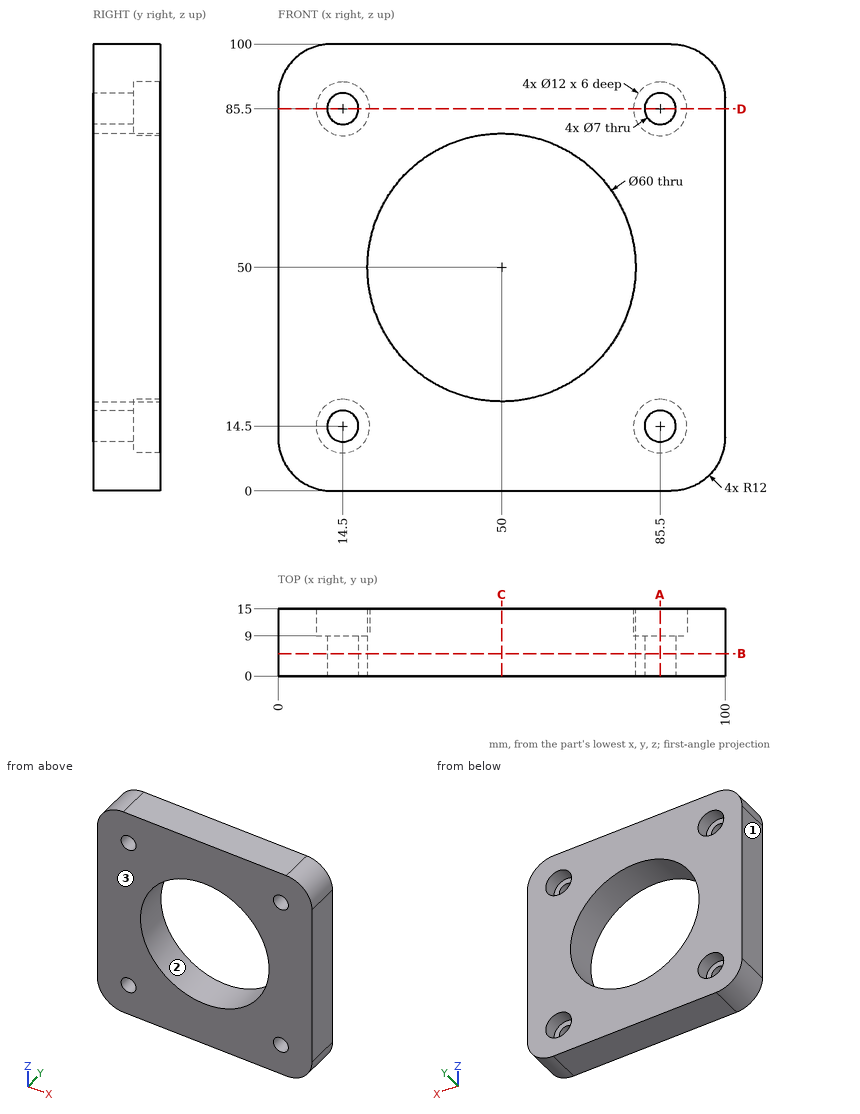
Study the drawing (mm; zero at the part's minimum x, y, z) and answer. Coordinates: 2 decimals unless noted, no trailing zeros. Write each loop counter-clockwise with the first axis right and the second up, starting at its lowest first coordinate (ties: lowest second). Pieces come first, ordered by that corner, then holes. Notation, with made-up numbers: (77.5, 62) - (127.5, 62) arc R16 ccw to (127.5, 89) - close; hole circle Ø3 at (70.5, 60.5). An arc over 180 degrees is marked (long way). One line per item, written item: value.
1) Consider line 1 along X through (y, z) = (10.9, 85.5); line 2 along X through (y, z) = (4.25, 14.5). Determine where each line is inside the solid, lowest interval first. Write a range as from..to.
Geometry check:
line 1: x = 0..8.5, 20.5..79.5, 91.5..100
line 2: x = 0..11, 18..82, 89..100
2) Find section D-D (z = 85.5). Give the vertices of the cut face in (x, y).
Geometry check:
outline: (0, 0) - (11, 0) - (11, 9) - (8.5, 9) - (8.5, 15) - (0, 15) - close; (18, 0) - (82, 0) - (82, 9) - (79.5, 9) - (79.5, 15) - (20.5, 15) - (20.5, 9) - (18, 9) - close; (89, 0) - (100, 0) - (100, 15) - (91.5, 15) - (91.5, 9) - (89, 9) - close
3) For a pull along X with two mould halves and no side action, classify the marked faces 1, 2 and 3 as pulls with the +X half, pulls with the -X half, needs draft (parallel to the pull), parting line crosses it, or undercut.
Geometry check:
face 1: pulls with the -X half
face 2: undercut
face 3: needs draft
4) Find section C-C (x = 50). Give the vertices of the cut face in (y, z).
Geometry check:
outline: (0, 0) - (15, 0) - (15, 20) - (0, 20) - close; (0, 80) - (15, 80) - (15, 100) - (0, 100) - close
5) Find section B-B (y = 5). Give the vertices of the cut face in (x, z), and give its area (4 significant figures).
Geometry check:
outline: (0, 12) arc R12 ccw to (12, 0) - (88, 0) arc R12 ccw to (100, 12) - (100, 88) arc R12 ccw to (88, 100) - (12, 100) arc R12 ccw to (0, 88) - close; hole circle Ø7 at (14.5, 14.5); hole circle Ø7 at (14.5, 85.5); hole circle Ø60 at (50, 50); hole circle Ø7 at (85.5, 14.5); hole circle Ø7 at (85.5, 85.5)
area: 6,895 mm2
6) Find section A-A (x = 85.5). Give the vertices of the cut face in (y, z).
Geometry check:
outline: (0, 0) - (15, 0) - (15, 8.5) - (9, 8.5) - (9, 11) - (0, 11) - close; (0, 18) - (9, 18) - (9, 20.5) - (15, 20.5) - (15, 79.5) - (9, 79.5) - (9, 82) - (0, 82) - close; (0, 89) - (9, 89) - (9, 91.5) - (15, 91.5) - (15, 100) - (0, 100) - close
7) This flat-tipped pin is pushed along its axis until it touches: pin 1 Ø3.5 at (x, z) = (83, 83) entering from +Y. Where does it stop, or does it pass through?
Geometry check:
pin 1: stops at y = 9
